Verification items for this drawing (mm, ordinates from the low corner). A direction names the side the tool comes from. Give positions to 0.01 mm unless a question says otherwise; leave off trailing zeros. Order: outer loops, then holes, each group sorted by start corner. A loop starts at its lowest first (then second) coordinate and runs counter-clockwise, first axis right, second up. Notation, with made-up numbers: M -17,-29.75 L -6,-29.75 A33 ccw -6,7.25 Z; hole C 87,-4.75 d1. An arc over 180 degrees is marked long. Answer as a JSON object with one key per item and string values.
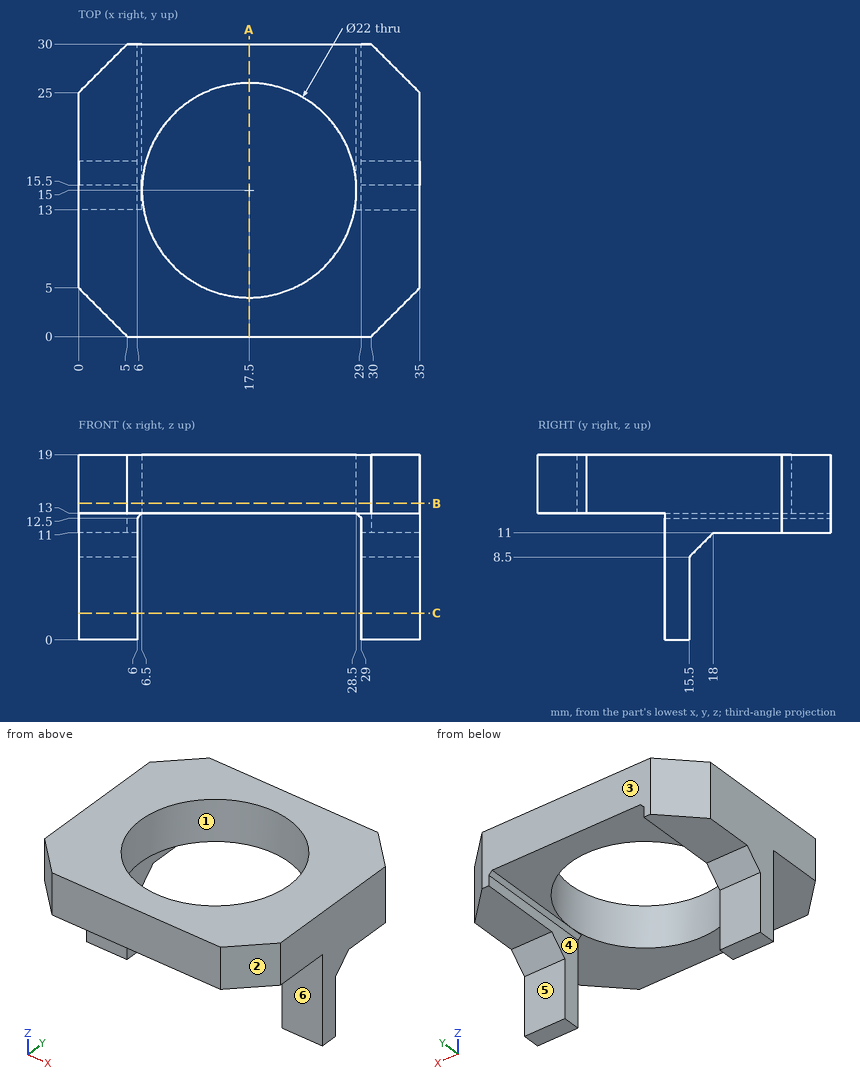
Q1. Release check for a two-part mould opening along Y. For the marked faces 1, 2 and 3 record: +Y half, -Y half, draft (parallel to the pull), parting line (faces both ways), or undercut.
Resolved:
{"face 1": "undercut", "face 2": "-Y half", "face 3": "+Y half"}
Q2. Gauge pin test, flat ends, axial feed: pin 1 Ø3 at (x, z) = (32, 2.5) entering from +Y; pin 2 Ø3 at (x, y) = (31.5, 23.5) entering from -Z; pin 3 Ø7 at (x, z) = (32.5, 7) entering from -Y. Record the tip position at first contact, or that the pin passes through.
Resolved:
{"pin 1": "stops at y = 15.5", "pin 2": "stops at z = 11", "pin 3": "stops at y = 13"}
Q3. Section check C-C on z = 2.75. Record the cut outline in (x, y).
Resolved:
{"outline": "M 0,13 L 6,13 L 6,15.5 L 0,15.5 Z; M 29,13 L 35,13 L 35,15.5 L 29,15.5 Z"}
Q4. Material ranges on L1, parallel to X at y = 14.5, z = 1; L2, parallel to Z at x = 25.5, y = 23; L3, parallel to Y at x = 17.5, z = 16.95, recorded low to high.
Resolved:
{"L1": "x = 0 to 6, 29 to 35", "L2": "z = 13 to 19", "L3": "y = 0 to 4, 26 to 30"}
Q5. Section check B-B on z = 14. Record the cut outline in (x, y), then the cut area to 3 significant figures.
Resolved:
{"outline": "M 0,5 L 5,0 L 30,0 L 35,5 L 35,25 L 30,30 L 5,30 L 0,25 Z; hole C 17.5,15 d22", "area": "620 mm²"}
Q6. Section check A-A on x = 17.5. Record the cut outline in (y, z), then the cut area to 3 significant figures.
Resolved:
{"outline": "M 0,13 L 4,13 L 4,19 L 0,19 Z; M 26,13 L 30,13 L 30,19 L 26,19 Z", "area": "48.0 mm²"}
Q7. Tool access check on the marked faces 4, 5 and 6. Record the directions out of +Z, -Z, +X, -X, +Y, -Y that give a thin tool (end or side, any length) a straight path to the whole face; none if there is none.
Resolved:
{"face 4": "-Z, +Y, -Y", "face 5": "-Z, +X, -X, +Y", "face 6": "-Z, +X, -X, -Y"}
